Here's how the part is built. I have some questions about the finished solid (model axes, mm). Face numbers are marked on the shaded views. A direction names the side the tool comes from. Round coordinates to 2 decimals unless told otherwise and drop trailing zeros. Order: outer loops, then holes, each group sorted by start corner. A loop starts at its lowest first (then second) coordinate and runs counter-clockwise, first axis right, second up. Notation, with made-up numbers: (14, -21) -> (61, -21) arc R20 ccw to (61, -14) -> close; hole circle Ø6 at (81, -30). An arc over 180 degrees is marked (long way). Answer in a Markdown table with one row per item.
```python
from build123d import *

# Parameters (mm, degrees)
F0_W          = 24
F0_H          = 24
F1_DEPTH      = 3.6
F2_R          = 4.3
F2_R_2        = 2.25
F3_DEPTH      = 4.5
F4_DEPTH      = 10
F5_R          = 2.25
F6_DEPTH      = 6.7
F7_W          = 17.1
F7_H          = 17.1
F7_R          = 2.25
F8_DEPTH      = 2
F9_W          = 17.1
F9_H          = 17.1
F9_R          = 2.25
F10_DEPTH     = 6.7
F11_W         = 17.1
F11_H         = 17.1
F11_R         = 2.25
F12_DEPTH     = 2
F13_W         = 17.1
F13_H         = 17.1
F14_DEPTH     = 6.7
F15_W         = 24
F15_H         = 24
F16_DEPTH     = 3.4
F17_R         = 5.1
F18_R         = 12
F19_R         = 4.1
F20_DEPTH     = 23
F23_DEPTH     = 25
F24_DEPTH     = 25
F25_DEPTH     = 50
F26_T1_DEPTH  = 14.1796577476
F26_T3_DEPTH  = 30.9358787863
F26_T5_DEPTH  = 30.9358787863
F26_T7_DEPTH  = 14.1796577476
F26_T10_ANGLE = 90
F27_R         = 2
F28_R         = 2
F29_R         = 2


# Not quite as in the source:
# - a fillet or chamfer that OpenCascade refuses, or shapes differently, is made with other operations: its cross-section is extruded or revolved along the edge and cut away or added


with BuildPart() as f1:
    # F0 (on Top) → F1 (new body)
    with BuildSketch(Plane.XY):
        with Locations((12, 12)):
            Rectangle(F0_W, F0_H)
    extrude(amount=F1_DEPTH)

    # F2 (on face) → F3 (join)
    with BuildSketch(Plane(origin=(0, 0, 0), x_dir=(1, 0, 0), z_dir=(0, 0, -1))):
        with Locations((12, -12)):
            Circle(F2_R)
        with Locations((12, -12)):
            Circle(F2_R_2, mode=Mode.SUBTRACT)
    extrude(amount=F3_DEPTH)

    # F4 (cut): a face of the model
    f4_faces = [f1.faces().sort_by_distance(p)[0] for p in [
        (12, 12, 0),
    ]]
    extrude(f4_faces, amount=-F4_DEPTH, mode=Mode.SUBTRACT)

    # F5 (on face) → F6 (join)
    with BuildSketch(Plane.XY.offset(3.6)):
        Polygon((6.9, 0), (20, 0), (24, 0), (24, 17.1), (6.9, 17.1), align=None)
        with Locations((12, 12)):
            Circle(F5_R, mode=Mode.SUBTRACT)
    extrude(amount=F6_DEPTH)

    # F7 (on face) → F8 (join)
    with BuildSketch(Plane.XY.offset(10.3)):
        Polygon((0, 24), (0, 0), (6.9, 0), (6.9, 17.1), (24, 17.1), (24, 24), align=None)
        with Locations((15.45, 8.55)):
            Rectangle(F7_W, F7_H)
        with Locations((12, 12)):
            Circle(F7_R, mode=Mode.SUBTRACT)
    extrude(amount=F8_DEPTH)

    # F9 (on face) → F10 (join)
    with BuildSketch(Plane.XY.offset(12.3)):
        with Locations((15.45, 8.55)):
            Rectangle(F9_W, F9_H)
        with Locations((12, 12)):
            Circle(F9_R, mode=Mode.SUBTRACT)
    extrude(amount=F10_DEPTH)

    # F11 (on face) → F12 (join)
    with BuildSketch(Plane.XY.offset(19)):
        Polygon((0, 0), (6.9, 0), (6.9, 17.1), (24, 17.1), (24, 24), (0, 24), align=None)
        with Locations((15.45, 8.55)):
            Rectangle(F11_W, F11_H)
        with Locations((12, 12)):
            Circle(F11_R, mode=Mode.SUBTRACT)
    extrude(amount=F12_DEPTH)

    # F13 (on face) → F14 (join)
    with BuildSketch(Plane.XY.offset(21)):
        with Locations((15.45, 8.55)):
            Rectangle(F13_W, F13_H)
    extrude(amount=F14_DEPTH)

    # F15 (on face) → F16 (join)
    with BuildSketch(Plane.XY.offset(27.7)):
        with Locations((12, 12)):
            Rectangle(F15_W, F15_H)
    extrude(amount=F16_DEPTH)

    # F17
    f17_edges = [f1.edges().sort_by_distance(p)[0] for p in [
        (6.9, 17.1, 6.95),
        (6.9, 17.1, 15.65),
        (6.9, 17.1, 24.35),
    ]]
    fillet(f17_edges, radius=F17_R)

    # F18
    f18_edges = [f1.edges().sort_by_distance(p)[0] for p in [
        (0, 24, 11.3),
        (0, 24, 20),
        (0, 24, 29.4),
    ]]
    fillet(f18_edges, radius=F18_R)

    # F19 (on face) → F20 (cut)
    with BuildSketch(Plane.XY.offset(31.1)):
        with Locations((12, 12)):
            Circle(F19_R)
    extrude(amount=-F20_DEPTH, mode=Mode.SUBTRACT)

    # F21 (on face) → F23 (join)
    with BuildSketch(Plane.YZ.offset(24)):
        Polygon((0, 31.1), (0, 0), (3, 31.1), align=None)
    extrude(amount=F23_DEPTH)

    # F22 (on face) → F24 (cut)
    with BuildSketch(Plane.XZ):
        Polygon((21, 31.1), (24, 0), (24, 31.1), align=None)
    extrude(amount=-F24_DEPTH, mode=Mode.SUBTRACT)

    # F25 (cut): a face of the model
    f25_faces = [f1.faces().sort_by_distance(p)[0] for p in [
        (49, 1, 20.7333333333),
    ]]
    extrude(f25_faces, amount=-F25_DEPTH, mode=Mode.SUBTRACT)

    # F26: chamfer of 1 x 2 on 5 edges, made by hand

    # F26_s2 → F26_t1 (cut)
    with BuildSketch(Plane.XZ.offset(-12)):
        Polygon((2, 31.1), (0, 30.1), (0, 31.1), align=None)
    extrude(amount=F26_T1_DEPTH, mode=Mode.SUBTRACT)

    # F26_s4 → F26_t3 (cut)
    with BuildSketch(Plane.YZ.offset(-4.9679393932)):
        Polygon((2.9220612214, 30.2920346615), (4.912820546, 31.1), (3, 31.1), align=None)
    extrude(amount=F26_T3_DEPTH, mode=Mode.SUBTRACT)

    # F26_s6 → F26_t5 (cut)
    with BuildSketch(Plane.XZ.offset(-28.9679393932)):
        Polygon((21.0779387786, 30.2920346615), (19.087179454, 31.1), (21, 31.1), align=None)
    extrude(amount=F26_T5_DEPTH, mode=Mode.SUBTRACT)

    # F26_s8 → F26_t7 (cut)
    with BuildSketch(Plane.YZ.offset(12)):
        Polygon((24, 30.1), (22, 31.1), (24, 31.1), align=None)
    extrude(amount=F26_T7_DEPTH, mode=Mode.SUBTRACT)

    # F26_s9 → F26_t10 (revolve, cut)
    with BuildSketch(Plane.YZ.offset(12)):
        Polygon((22, 31.1), (24, 30.1), (24, 31.1), align=None)
    revolve(axis=Axis((12, 12, 31.1), (0, 0, 1)), revolution_arc=F26_T10_ANGLE, mode=Mode.SUBTRACT)

    # F27
    f27_edges = [f1.edges().sort_by_distance(p)[0] for p in [
        (22.538969, 1.461031, 15.146017),
    ]]
    fillet(f27_edges, radius=F27_R)

    # F28
    f28_edges = [f1.edges().sort_by_distance(p)[0] for p in [
        (0, 2.787781, 28.9),
        (0, 1.92926, 20),
        (0, 1.090032, 11.3),
        (0, 0.173633, 1.8),
        (0, 24, 1.8),
        (23.826367, 24, 1.8),
        (22.909968, 24, 11.3),
        (22.07074, 24, 20),
        (21.212219, 24, 28.9),
    ]]
    fillet(f28_edges, radius=F28_R)

    # F29
    f29_edges = [f1.edges().sort_by_distance(p)[0] for p in [
        (7.7, 12, -4.5),
    ]]
    fillet(f29_edges, radius=F29_R)


solid = f1.part
```
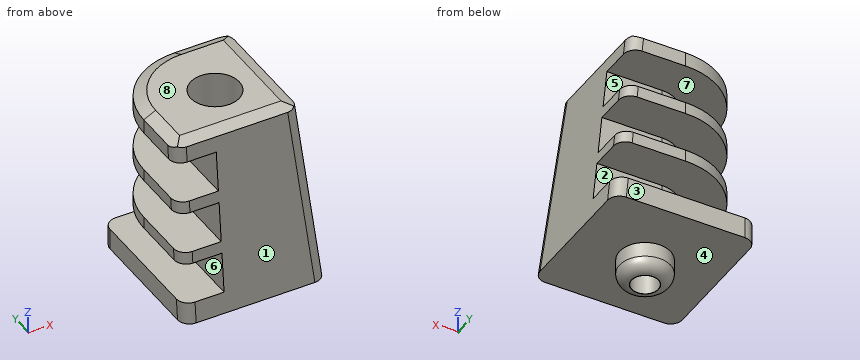
1. For the marked faces 4, 5, 6, 7 and 8, which set-ups out of +Z, -Z, +X, -X, +Y, -Y let a thin tool reach every point of the face, with its end or its side?
Numbers:
| item | result |
|---|---|
| face 4 | -Z |
| face 5 | +X, -X, +Y |
| face 6 | -X, +Y, -Y |
| face 7 | -X, +Y |
| face 8 | +Z, +X, -X, +Y, -Y |
2. Suppose I cut it at A-A on x = 18. Write out the boundary of the cut face in (y, z).
Numbers:
| item | result |
|---|---|
| outline | (0, 0) -> (24, 0) -> (24, 3.6) -> (17.1, 3.6) -> (17.1, 10.3) -> (24, 10.3) -> (24, 12.3) -> (17.1, 12.3) -> (17.1, 19) -> (24, 19) -> (24, 21) -> (17.1, 21) -> (17.1, 27.7) -> (24, 27.7) -> (24, 30.1) -> (22, 31.1) -> (4.91, 31.1) -> (2.92, 30.29) -> close |
3. Please list where these lines run through material, in increasing order: line 1 along Z through (x, y) = (14.25, 17.25); line 2 along Y through (x, z) = (12, 3.5); line 3 along Y through (x, z) = (12, -2).
Numbers:
| item | result |
|---|---|
| line 1 | z = 0 to 3.6, 10.3 to 12.3, 19 to 21, 27.7 to 31.1 |
| line 2 | y = 0.34 to 9.75, 14.25 to 24 |
| line 3 | y = 7.7 to 9.75, 14.25 to 16.3 |
4. For pin 1 Ø4 at (x, z) = (3.5, 10.5) entering from +Y; pin 2 Ø7.5 at (y, z) = (3.5, 6) entering from -X; pin 3 Ø10 at (y, z) = (9, 24.5) entering from +X; pin 4 Ø4 at (x, y) = (3, 8) entering from -Z, each with a flat end and sliding along its axis, tell me the tip position at first contact or that it passes through.
Numbers:
| item | result |
|---|---|
| pin 1 | stops at y = 22.09 |
| pin 2 | stops at x = 0 |
| pin 3 | stops at x = 22.12 |
| pin 4 | stops at z = 0 |
5. We'd pull the mould along Z, two halves only. Please class the marked faces 1, 2 and 3: released by +Z, released by -Z, zero draft, split by the parting line, or undercut.
Numbers:
| item | result |
|---|---|
| face 1 | released by +Z |
| face 2 | undercut |
| face 3 | zero draft |
6. Suppose I cut it at B-B on x = 5.75. State how many separate pieces and enclosed holes the cut face has, then the cut area to 3 significant figures.
Numbers:
| item | result |
|---|---|
| separate pieces | 4 |
| enclosed holes | 0 |
| area | 233 mm2 |
